For this review, take the finished solid that the model builds, in its own axes (mm). A direction names the side the tool comes from. Give positions to 0.01 mm unless a question says otherwise; leave off trailing zeros. Write each loop counter-clockwise with the first axis right and the second up, starting at its lowest first coordinate (ties: lowest second). Pieces come first, ordered by that corner, then holes.
1) Machinability: for faces 1 (the face through (10.2, -2, 1)), 2 (the face through (3.5, 3.75, -1.6)), 3 (the face through (0, 0, 8.6)), 4 (the face through (3.5, 4.75, -1.6)), 5 (the face through (4, 4, -2)), which of the approach directions +Z, -Z, +X, -X, +Y, -Y give a long, thin tool a straight path to every point of the face, cutting with its end or side? Answer none if there is none.
2) Draft analysis for pull direction X (two halves, no side actions). For faces 6 (the face through (-10, 4, -2)), 7 (the face through (-7, 3.75, -2)), state which applies: pulls with the +X half, pulls with the -X half, needs draft (parallel to the pull), parting line crosses it, or undercut.
3) We need section D-D on z = 1. Give the boundary of the cut face in (x, y).
4) For P1, Ø1.5, axis at x = 10, y = -2, coming from the -Z side; P2, Ø3, axis at x = 5.5, z = -2, coming from the +Y side; P3, Ø0.5, axis at y = 4.5, z = -2, coming from the +X side, all flat-tipped, find the tip position at first contact; note any pin that passes through.
5) We need section B-B on z = -1.75. Give the boundary of the cut face in (x, y), and give its area (3 significant figures).
6) We need section C-C on x = -5.75. Give the boundary of the cut face in (y, z).
7) Wall thickness on line 1 along X through (y, z) = (-3.75, 0.25); line 2 along X through (y, z) = (-2.5, 5.25); line 3 along Z through (x, y) = (-11.5, 1): over which ranges is each line inside the solid? List them lowest first.
8) We need section A-A on y = -3. Give the boundary of the cut face in (x, z).
from build123d import *

# Parameters (mm, degrees)
SKETCH_1_W                         = 26.8
SKETCH_1_H                         = 10.5
EXTRUDE_1_DEPTH                    = 8.6
CUT_EXTRUDE_1_DEPTH                = 7
EXTRUDE_START                      = -5
SKETCH_3_W                         = 1
SKETCH_3_H                         = 1
EXTRUDE_2_DEPTH                    = 8.6
CHAMFER_1_SIZE                     = 0.3
PATTERN_LINEAR_1_COUNT             = 7
PATTERN_LINEAR_1_PITCH             = 3.5
CHAMFER_1_OF_PATTERN_LINEAR_1_SIZE = 0.3


with BuildPart() as part:
    # Эскиз1 → Бобышка-Вытянуть1 (new body)
    with BuildSketch(Plane.XY):
        Rectangle(SKETCH_1_W, SKETCH_1_H)
    extrude(amount=EXTRUDE_1_DEPTH)

    # Эскиз2 → Вырез-Вытянуть1 (cut)
    with BuildSketch(Plane.XZ.offset(5.25)):
        Polygon((-12.4, 6.6), (12.4, 6.6), (12.4, 0.2), (10.2, 0.2), (10.2, 1.8), (-8.6, 1.8), (-8.6, 0.2), (-10.8, 0.2), (-10.8, 1.8), (-12.4, 1.8), align=None)
    extrude(amount=-CUT_EXTRUDE_1_DEPTH, mode=Mode.SUBTRACT)

    # Эскиз3 → Бобышка-Вытянуть2 (add)
    with BuildSketch(Plane(origin=(0, 0, 0), x_dir=(-1, 0, 0), z_dir=(0, 0, -1)).offset(EXTRUDE_START)):
        with Locations((10.5, 4.25)):
            Rectangle(SKETCH_3_W, SKETCH_3_H)
    extrude_2 = extrude(amount=EXTRUDE_2_DEPTH)

    # Фаска1
    chamfer_1_edges = [part.edges().sort_by_distance(p)[0] for p in [
        (-10, 4.25, -3.6),
        (-10.5, 3.75, -3.6),
        (-11, 4.25, -3.6),
        (-10.5, 4.75, -3.6),
    ]]
    chamfer(chamfer_1_edges, length=CHAMFER_1_SIZE)

    # Линейный массив1: Бобышка-Вытянуть2 ×7
    with Locations(*[(i * PATTERN_LINEAR_1_PITCH, 0, 0) for i in range(1, PATTERN_LINEAR_1_COUNT)]):
        add(extrude_2)

    # Фаска1 of Линейный массив1
    chamfer_1_of_pattern_linear_1_edges = [part.edges().sort_by_distance(p)[0] for p in [
        (-6.5, 4.25, -3.6),
        (-7, 3.75, -3.6),
        (-7.5, 4.25, -3.6),
        (-7, 4.75, -3.6),
        (-3, 4.25, -3.6),
        (-3.5, 3.75, -3.6),
        (-4, 4.25, -3.6),
        (-3.5, 4.75, -3.6),
        (0.5, 4.25, -3.6),
        (0, 3.75, -3.6),
        (-0.5, 4.25, -3.6),
        (0, 4.75, -3.6),
        (4, 4.25, -3.6),
        (3.5, 3.75, -3.6),
        (3, 4.25, -3.6),
        (3.5, 4.75, -3.6),
        (7.5, 4.25, -3.6),
        (7, 3.75, -3.6),
        (6.5, 4.25, -3.6),
        (7, 4.75, -3.6),
        (11, 4.25, -3.6),
        (10.5, 3.75, -3.6),
        (10, 4.25, -3.6),
        (10.5, 4.75, -3.6),
    ]]
    chamfer(chamfer_1_of_pattern_linear_1_edges, length=CHAMFER_1_OF_PATTERN_LINEAR_1_SIZE)


solid = part.part
Results list:
1. face 1: -Y
1. face 2: -Z, +X, -X, -Y
1. face 3: +Z, +X, -X, +Y, -Y
1. face 4: -Z, +X, -X, +Y
1. face 5: -Z, +Y, -Y
2. face 6: undercut
2. face 7: needs draft
3. outline: (-13.4, -5.25) - (-10.8, -5.25) - (-10.8, 1.75) - (-8.6, 1.75) - (-8.6, -5.25) - (10.2, -5.25) - (10.2, 1.75) - (12.4, 1.75) - (12.4, -5.25) - (13.4, -5.25) - (13.4, 5.25) - (-13.4, 5.25) - close
4. P1: stops at z = 0
4. P2: stops at y = 4.75
4. P3: stops at x = 11
5. outline: (-11, 3.75) - (-10, 3.75) - (-10, 4.75) - (-11, 4.75) - close; (-7.5, 3.75) - (-6.5, 3.75) - (-6.5, 4.75) - (-7.5, 4.75) - close; (-4, 3.75) - (-3, 3.75) - (-3, 4.75) - (-4, 4.75) - close; (-0.5, 3.75) - (0.5, 3.75) - (0.5, 4.75) - (-0.5, 4.75) - close; (3, 3.75) - (4, 3.75) - (4, 4.75) - (3, 4.75) - close; (6.5, 3.75) - (7.5, 3.75) - (7.5, 4.75) - (6.5, 4.75) - close; (10, 3.75) - (11, 3.75) - (11, 4.75) - (10, 4.75) - close
5. area: 7.00 mm2
6. outline: (-5.25, 0) - (5.25, 0) - (5.25, 8.6) - (-5.25, 8.6) - (-5.25, 6.6) - (1.75, 6.6) - (1.75, 1.8) - (-5.25, 1.8) - close
7. line 1: x = -13.4 to -10.8, -8.6 to 10.2, 12.4 to 13.4
7. line 2: x = -13.4 to -12.4, 12.4 to 13.4
7. line 3: z = 0 to 1.8, 6.6 to 8.6
8. outline: (-13.4, 0) - (13.4, 0) - (13.4, 8.6) - (-13.4, 8.6) - close; hole (-12.4, 1.8) - (-10.8, 1.8) - (-10.8, 0.2) - (-8.6, 0.2) - (-8.6, 1.8) - (10.2, 1.8) - (10.2, 0.2) - (12.4, 0.2) - (12.4, 6.6) - (-12.4, 6.6) - close
